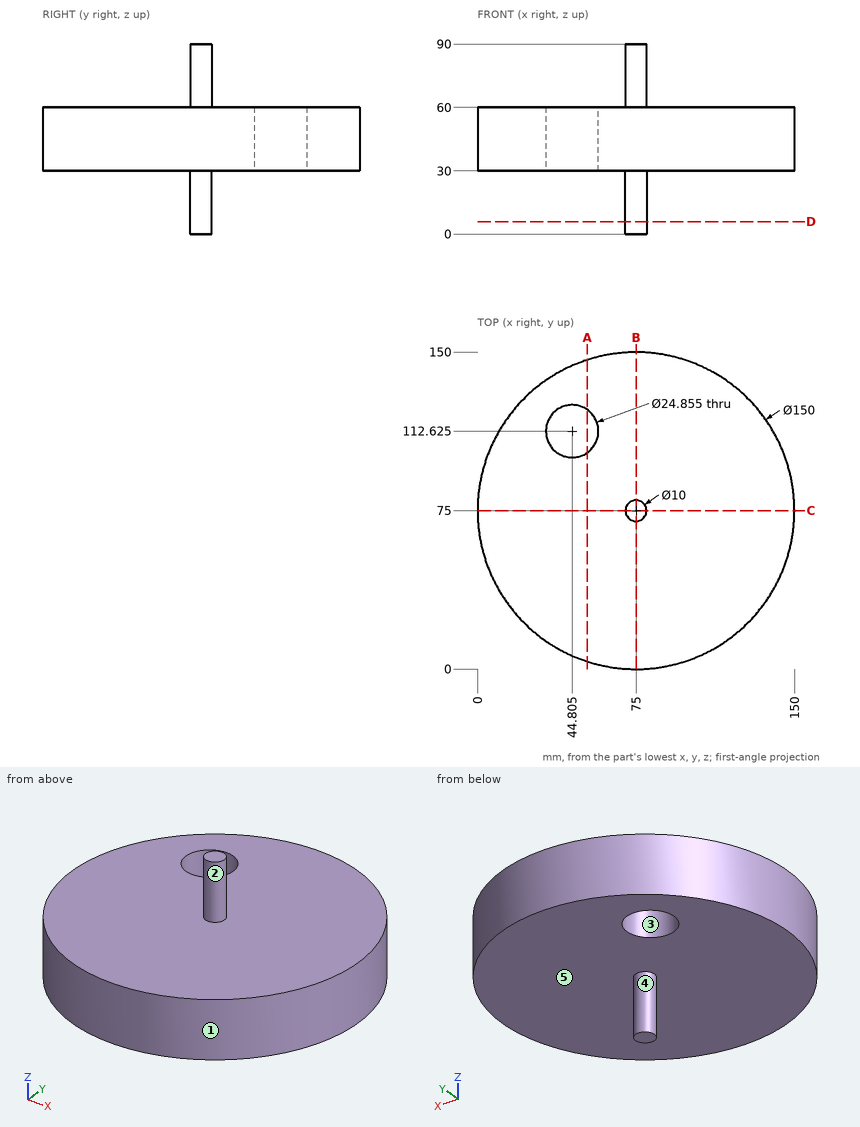
Design review of the part shown in the three views and the two pictorial views. Dimensions are in mm from the part's minimum x, y and z. A direction names the side the tool comes from. Give positions to 0.01 mm unless a question says otherwise; leave off trailing zeros. Write each loop counter-clockwise with the first axis right and the second up, starting at its lowest first coordinate (ties: lowest second). Pieces come first, ordered by that corner, then holes.
(1) Add section D-D (z = 6). Give the boundary of the cut face in (x, y).
Checked values:
outline: circle Ø10 at (75, 75)
(2) Tool access review of the marked faces 1 and 2: name each direction out of +Z, -Z, +X, -X, +Y, -Y from which nothing blocks a thin tool from reaching the whole face with its end or side.
Checked values:
face 1: +Z, -Z
face 2: +Z
(3) Add section B-B (x = 75). Give the boundary of the cut face in (y, z).
Checked values:
outline: (0, 30) - (70, 30) - (70, 0) - (80, 0) - (80, 30) - (150, 30) - (150, 60) - (80, 60) - (80, 90) - (70, 90) - (70, 60) - (0, 60) - close
(4) Wall thickness on line 1 along Z through (x, y) = (25.5, 105.5); line 2 along X through (y, z) = (76, 59.5); line 3 along Y through (x, z) = (67.5, 42.5) (1 decimal): over which ranges is each line inside the solid? List them lowest first.
Checked values:
line 1: z = 30 to 60
line 2: x = 0.01 to 149.99
line 3: y = 0.4 to 149.6
(5) Add section A-A (x = 52). Give the boundary of the cut face in (y, z).
Checked values:
outline: (3.61, 30) - (102.49, 30) - (102.49, 60) - (3.61, 60) - close; (122.76, 30) - (146.39, 30) - (146.39, 60) - (122.76, 60) - close
(6) Mouldability with a two-part tool opening along Y and no side actions: class the marked faces 3, 4 and 5 as +Y half, -Y half, draft (parallel to the pull), parting line (faces both ways), or undercut.
Checked values:
face 3: undercut
face 4: parting line
face 5: draft
(7) Clearance check with flat-ended pins moving along their axes: pin 1 Ø6 at (x, z) = (133.5, 52.5) entering from -Y (1 decimal); pin 2 Ø12 at (x, z) = (38, 56) entering from -Y; pin 3 Ø22.5 at (x, y) = (44.8, 112.63) entering from -Z; pin 4 Ø5 at (x, y) = (34.5, 126.5) entering from +Z. State where each tip first meets the part, or that it passes through.
Checked values:
pin 1: stops at y = 24.6
pin 2: stops at y = 6.71
pin 3: passes through
pin 4: stops at z = 60
